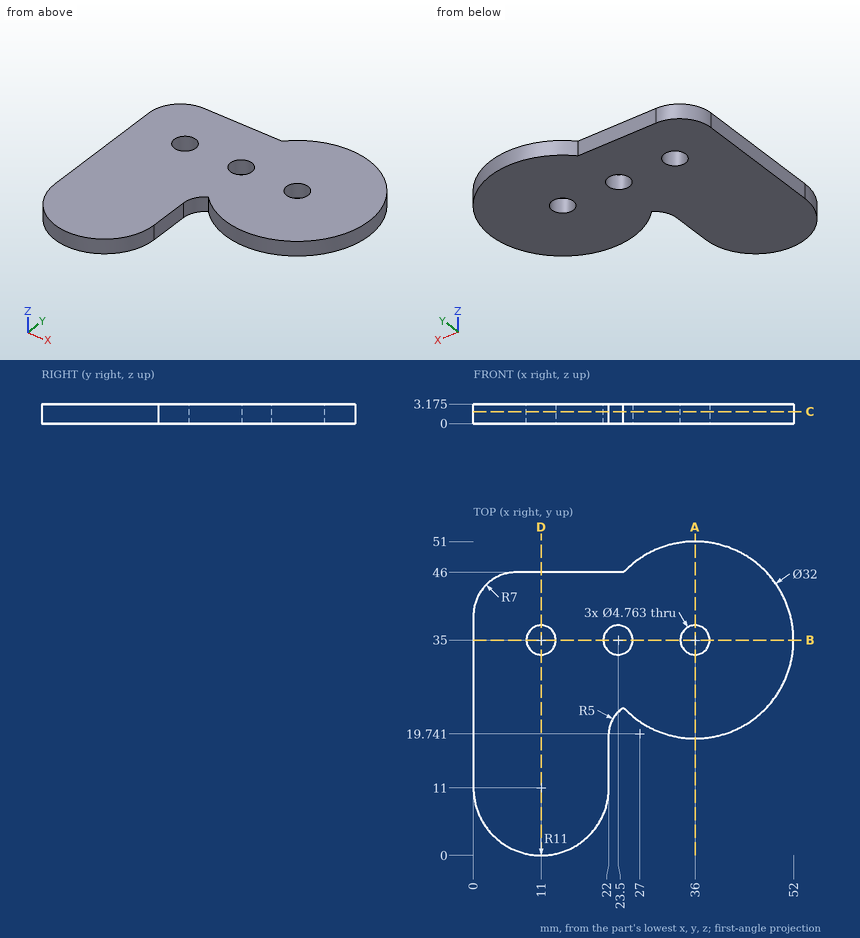
For this review, use the dimensioned drawing (mm, ordinates from the lowest corner) and the shaded views. Round coordinates to 2 decimals unless told otherwise and drop trailing zeros. Write each loop counter-clockwise with the first axis right and the second up, starting at its lowest first coordinate (ties: lowest second). Pieces come first, ordered by that corner, then holes. Notation, with made-up numbers: (17.25, 67) -> (58.25, 67) arc R24 cw to (58.25, 86) -> close; hole circle Ø1 at (-20.5, 52). An arc over 180 degrees is marked (long way). Use CSV: the item, a comma, the result in double quotes.
(1) Consider section A-A, the plane x = 36. Give the boundary of the cut face in (y, z) (1 decimal).
Computed values:
outline,"(19, 0) -> (32.6, 0) -> (32.6, 3.2) -> (19, 3.2) -> close; (37.4, 0) -> (51, 0) -> (51, 3.2) -> (37.4, 3.2) -> close"
(2) Consider section B-B, the plane y = 35. Give the boundary of the cut face in (x, z) (1 decimal).
Computed values:
outline,"(0, 0) -> (8.6, 0) -> (8.6, 3.2) -> (0, 3.2) -> close; (13.4, 0) -> (21.1, 0) -> (21.1, 3.2) -> (13.4, 3.2) -> close; (25.9, 0) -> (33.6, 0) -> (33.6, 3.2) -> (25.9, 3.2) -> close; (38.4, 0) -> (52, 0) -> (52, 3.2) -> (38.4, 3.2) -> close"
(3) Clearance check with a flat-ended pin moving along its axis: P1, Ø1.6, axis at x = 15.5, z = 2, coming from the +Y side. State where the tip first meets the part, or that it passes through.
Computed values:
P1,"y = 46"
(4) Consider section D-D, the plane x = 11. Give the boundary of the cut face in (y, z) (1 decimal), plus the area to 3 significant figures.
Computed values:
outline,"(0, 0) -> (32.6, 0) -> (32.6, 3.2) -> (0, 3.2) -> close; (37.4, 0) -> (46, 0) -> (46, 3.2) -> (37.4, 3.2) -> close"
area,"131 mm²"
(5) To check wall thickness, follow L1, parallel to Y at x = 11, z = 0.7; L2, parallel to X at y = 23, z = 1.95 (1 decimal); L3, parallel to X at y = 17, z = 1.9. State the ranges of each line that lie inside material, in increasing order. Write a range as [from, to].
Computed values:
L1,"[0, 32.62], [37.38, 46]"
L2,"[0, 23.2], [25.4, 46.6]"
L3,"[0, 22]"
(6) Consider section C-C, the plane z = 1.95. Give the boundary of the cut face in (x, y), plus the area to 3 significant figures.
Computed values:
outline,"(0, 11) arc R11 ccw to (22, 11) -> (22, 19.74) arc R5 cw to (24.38, 24) arc R16 ccw (long way) to (24.38, 46) -> (7, 46) arc R7 ccw to (0, 39) -> close; hole circle Ø4.76 at (11, 35); hole circle Ø4.76 at (23.5, 35); hole circle Ø4.76 at (36, 35)"
area,"1,690 mm²"
